from build123d import *

# Parameters (mm, degrees)
F0_W           = 50
F0_H           = 50
F1_DEPTH       = 25
F3_D           = 5.2
F3_CBORE_D     = 10
F3_CBORE_DEPTH = 5


with BuildPart() as f1:
    # F0 (on Top) → F1 (new body)
    with BuildSketch(Plane.XY):
        Rectangle(F0_W, F0_H)
    extrude(amount=-F1_DEPTH)

    # F3 (through all)
    with Locations(Plane.XY):
        with Locations((-15.721669, 16.288219)):
            CounterBoreHole(F3_D / 2, F3_CBORE_D / 2, F3_CBORE_DEPTH)


solid = f1.part
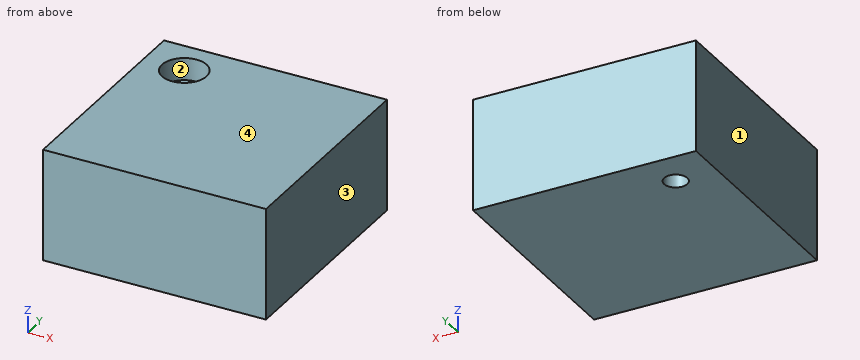
CAD build for the part. Positions are in the model's coordinates, mm. Face numbers are marked on the shaded views. Round coordinates to 2 decimals unless told otherwise and drop trailing zeros. Loops run counter-clockwise (first coordinate to the right, second up) from the corner with the lowest first, then second, coordinate; pieces in that order, holes last.
(1) Two-plate mould, pull along X, no slides. Class the marked faces 1, 2, 3 and 4: +X half, -X half, draft (parallel to the pull), parting line (faces both ways), or undercut.
(2) Wall check: line 1 along Y through (x, z) = (-17.5, -12.5); line 2 along Y through (x, z) = (-17, -14.5). Give the ranges that are in metal, low to high.
(3) Cut at A-A (x = -14). Give the cut face in (y, z), plus the area to 3 significant figures.
(4) Cut at B-B (y = 20). Give the cut face in (x, z).
(5) Drop a flat-ended pin along its axis: pin 1 (8.5 mm diameter, centred on x = -15.72, y = 16.29, fed in from +Z). Give the stop position or say it passes through.
Findings below:
1. face 1: -X half
1. face 2: undercut
1. face 3: +X half
1. face 4: draft
2. line 1: y = -25 to 14.39, 18.18 to 25
2. line 2: y = -25 to 14.02, 18.55 to 25
3. outline: (-25, -25) - (14.34, -25) - (14.34, -5) - (11.59, -5) - (11.59, 0) - (-25, 0) - close; (18.24, -25) - (25, -25) - (25, 0) - (20.98, 0) - (20.98, -5) - (18.24, -5) - close
3. area: 1,130 mm2
4. outline: (-25, -25) - (25, -25) - (25, 0) - (-12.37, 0) - (-12.37, -5) - (-19.07, -5) - (-19.07, 0) - (-25, 0) - close
5. pin 1: stops at z = -5
